Verification items for the finished model (mm, model axes). Face numbers are marked on the shaded views. Give positions to 0.01 mm unless a question says otherwise; leave off trailing zeros. Order: outer loops, then holes, each group sorted by start corner. A loop starts at its lowest first (then second) coordinate and runs counter-clockwise, first axis right, second up.
from build123d import *

# Parameters (mm, degrees)
BOSS_EXTRUDE1_DEPTH = 50
CUT_EXTRUDE2_START  = -63.5
SKETCH3_W           = 20
SKETCH3_H           = 10
CUT_EXTRUDE2_DEPTH  = 64.5
SKETCH4_W           = 17.5
SKETCH4_H           = 7
CUT_EXTRUDE3_DEPTH  = 10
BOSS_EXTRUDE2_DEPTH = 10
CUT_EXTRUDE6_DEPTH  = 10
SKETCH16_R          = 1.5
CUT_EXTRUDE7_DEPTH  = 10
SKETCH17_R          = 1.5
CUT_EXTRUDE8_DEPTH  = 10
CUT_EXTRUDE9_START  = -10
SKETCH18_R          = 1.5
CUT_EXTRUDE9_DEPTH  = 137
SKETCH19_R          = 1.5
CUT_EXTRUDE10_DEPTH = 10


with BuildPart() as part:
    # Sketch1 → Boss-Extrude1 (new body)
    with BuildSketch(Plane.XY):
        with BuildLine():
            ThreePointArc((59.5, 0), (0, -59.5), (-59.5, 0))
            Line((-59.5, 0), (-62.5, 0))
            ThreePointArc((-62.5, 0), (0, -62.5), (62.5, 0))
            Line((62.5, 0), (59.5, 0))
        make_face()
    extrude(amount=BOSS_EXTRUDE1_DEPTH)

    # Sketch3 → Cut-Extrude2 (cut)
    with BuildSketch(Plane(origin=(0, 0, 0), x_dir=(1, 0, 0), z_dir=(0, 1, 0)).offset(CUT_EXTRUDE2_START)):
        with Locations((-52.5, -45)):
            Rectangle(SKETCH3_W, SKETCH3_H)
        with Locations((52.5, -45)):
            Rectangle(SKETCH3_W, SKETCH3_H)
    cut_extrude2 = extrude(amount=CUT_EXTRUDE2_DEPTH, mode=Mode.SUBTRACT)

    # Sketch4 → Cut-Extrude3 (cut)
    with BuildSketch(Plane.XY.offset(50)):
        with Locations((0, -62.5)):
            Rectangle(SKETCH4_W, SKETCH4_H)
    cut_extrude3 = extrude(amount=-CUT_EXTRUDE3_DEPTH, mode=Mode.SUBTRACT)

    # Sketch9 → Boss-Extrude2 (add)
    with BuildSketch(Plane.XY):
        with BuildLine():
            Line((-52.112697755, -24.30055005), (-55.284775009, -25.779713966))
            ThreePointArc((-55.284775009, -25.779713966), (-51.730933866, -32.325075118), (-47.405903649, -38.388543854))
            Line((-47.405903649, -38.388543854), (-44.685892784, -36.185922485))
            ThreePointArc((-44.685892784, -36.185922485), (-48.762765529, -30.470357693), (-52.112697755, -24.30055005))
        make_face()
        with BuildLine():
            ThreePointArc((47.405903649, -38.388543854), (51.730933866, -32.325075118), (55.284775009, -25.779713966))
            Line((55.284775009, -25.779713966), (52.112697755, -24.30055005))
            ThreePointArc((52.112697755, -24.30055005), (48.762765529, -30.470357693), (44.685892784, -36.185922485))
            Line((44.685892784, -36.185922485), (47.405903649, -38.388543854))
        make_face()
        with BuildLine():
            Line((-7.007487246, -57.071403719), (-7.434029948, -60.54531525))
            ThreePointArc((-7.434029948, -60.54531525), (0, -61), (7.434029948, -60.54531525))
            Line((7.434029948, -60.54531525), (7.007487246, -57.071403719))
            ThreePointArc((7.007487246, -57.071403719), (0, -57.5), (-7.007487246, -57.071403719))
        make_face()
    boss_extrude2 = extrude(amount=BOSS_EXTRUDE2_DEPTH)

    # Sketch15 → Cut-Extrude6 (cut)
    with BuildSketch(Plane.XY):
        with BuildLine():
            Line((-52.112697755, -24.30055005), (-55.284775009, -25.779713966))
            ThreePointArc((-55.284775009, -25.779713966), (-51.730933866, -32.325075118), (-47.405903649, -38.388543854))
            Line((-47.405903649, -38.388543854), (-44.685892784, -36.185922485))
            ThreePointArc((-44.685892784, -36.185922485), (-48.762765529, -30.470357693), (-52.112697755, -24.30055005))
        make_face()
        with BuildLine():
            Line((-7.007487246, -57.071403719), (-7.434029948, -60.54531525))
            ThreePointArc((-7.434029948, -60.54531525), (0, -61), (7.434029948, -60.54531525))
            Line((7.434029948, -60.54531525), (7.007487246, -57.071403719))
            ThreePointArc((7.007487246, -57.071403719), (0, -57.5), (-7.007487246, -57.071403719))
        make_face()
        with BuildLine():
            ThreePointArc((47.405903649, -38.388543854), (51.730933866, -32.325075118), (55.284775009, -25.779713966))
            Line((55.284775009, -25.779713966), (52.112697755, -24.30055005))
            ThreePointArc((52.112697755, -24.30055005), (48.762765529, -30.470357693), (44.685892784, -36.185922485))
            Line((44.685892784, -36.185922485), (47.405903649, -38.388543854))
        make_face()
    cut_extrude6 = extrude(amount=CUT_EXTRUDE6_DEPTH, mode=Mode.SUBTRACT)

    # Sketch16 → Cut-Extrude7 (cut, symmetric)
    with BuildSketch(Plane(origin=(-28.846172405, -52.039872575, 0), x_dir=(0.874619707, -0.48480962, 0), z_dir=(0.48480962, 0.874619707, 0))):
        with Locations((-0.663731696, -45)):
            Circle(SKETCH16_R)
    cut_extrude7 = extrude(amount=CUT_EXTRUDE7_DEPTH, both=True, mode=Mode.SUBTRACT)

    # Sketch17 → Cut-Extrude8 (cut, symmetric)
    with BuildSketch(Plane(origin=(28.846172405, -52.039872575, 0), x_dir=(0.874619707, 0.48480962, 0), z_dir=(-0.48480962, 0.874619707, 0))):
        with Locations((0.663731696, -45)):
            Circle(SKETCH17_R)
    cut_extrude8 = extrude(amount=CUT_EXTRUDE8_DEPTH, both=True, mode=Mode.SUBTRACT)

    # Sketch18 → Cut-Extrude9 (cut)
    with BuildSketch(Plane(origin=(59.5, 0, 0), x_dir=(0, 1, 0), z_dir=(-1, 0, 0)).offset(CUT_EXTRUDE9_START)):
        with Locations((-6, -31)):
            Circle(SKETCH18_R)
    cut_extrude9 = extrude(amount=CUT_EXTRUDE9_DEPTH, mode=Mode.SUBTRACT)

    # Sketch19 → Cut-Extrude10 (cut, symmetric)
    with BuildSketch(Plane(origin=(0, -59.5, 0), x_dir=(1, 0, 0), z_dir=(0, 1, 0))):
        with Locations((0, -31)):
            Circle(SKETCH19_R)
    cut_extrude10 = extrude(amount=CUT_EXTRUDE10_DEPTH, both=True, mode=Mode.SUBTRACT)

    # Mirror4: Cut-Extrude2, Cut-Extrude3, Boss-Extrude2, Cut-Extrude6, Cut-Extrude7, Cut-Extrude8, Cut-Extrude9, Cut-Extrude10 across plane
    add(cut_extrude2.mirror(Plane.XY.offset(25)), mode=Mode.SUBTRACT)
    add(cut_extrude3.mirror(Plane.XY.offset(25)), mode=Mode.SUBTRACT)
    add(boss_extrude2.mirror(Plane.XY.offset(25)))
    add(cut_extrude6.mirror(Plane.XY.offset(25)), mode=Mode.SUBTRACT)
    add(cut_extrude7.mirror(Plane.XY.offset(25)), mode=Mode.SUBTRACT)
    add(cut_extrude8.mirror(Plane.XY.offset(25)), mode=Mode.SUBTRACT)
    add(cut_extrude9.mirror(Plane.XY.offset(25)), mode=Mode.SUBTRACT)
    add(cut_extrude10.mirror(Plane.XY.offset(25)), mode=Mode.SUBTRACT)


solid = part.part
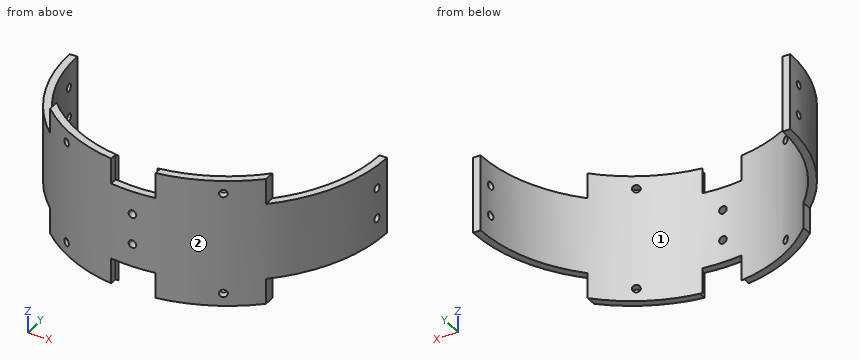
(1) Scan lines: line 1 (Z direction, x = 61.45, y = -6); line 2 (X direction, y = -30.5, z = 38.5); line 3 (X direction, y = -4, z = 25). Record each from-to range of solid material in increasing order.
Solved:
line 1: z = 10 to 17.5, 20.5 to 29.5, 32.5 to 40
line 2: x = -54.55 to -51.09, 51.09 to 54.55
line 3: x = -62.37 to -59.37, 59.37 to 62.37
(2) Go/stop test with flat-tipped pins: pin 1 (8 mm diameter, centred on x = -11, z = 30, fed in from +Y); pin 2 (5 mm diameter, centred on x = -5, z = 26, fed in from -Y); pin 3 (4 mm diameter, centred on y = -55.5, z = 13, fed in from -X); pin 4 (2.5 mm diameter, centred on x = 0, z = 19, fed in from -Y). Record where each tip stops, or that it passes through.
Solved:
pin 1: stops at y = -57.58
pin 2: stops at y = -62.45
pin 3: stops at x = -32.31
pin 4: passes through
(3) Section check D-D, the plane y = -44. Enter the section's corners in (x, z), then the cut area to 3 significant figures.
Solved:
outline: (-44.39, 10) - (-42.5, 10) - (-42.5, 0) - (-40.05, 0) - (-40.05, 50) - (-42.5, 50) - (-42.5, 40) - (-44.39, 40) - close; (40.05, 0) - (42.5, 0) - (42.5, 10) - (44.39, 10) - (44.39, 40) - (42.5, 40) - (42.5, 50) - (40.05, 50) - close
area: 358 mm2
(4) Section check C-C, the plane y = -6. Enter the section's corners in (x, z).
Solved:
outline: (-62.21, 10) - (-59.2, 10) - (-59.2, 17.5) - (-62.21, 17.5) - close; (-62.21, 20.5) - (-59.2, 20.5) - (-59.2, 29.5) - (-62.21, 29.5) - close; (-62.21, 32.5) - (-59.2, 32.5) - (-59.2, 40) - (-62.21, 40) - close; (59.2, 10) - (62.21, 10) - (62.21, 17.5) - (59.2, 17.5) - close; (59.2, 20.5) - (62.21, 20.5) - (62.21, 29.5) - (59.2, 29.5) - close; (59.2, 32.5) - (62.21, 32.5) - (62.21, 40) - (59.2, 40) - close
(5) Section check B-B, the plane z = 19. Enter the section's corners in (x, y).
Solved:
outline: (-62.5, 0) arc R62.5 ccw to (-62.34, -4.5) - (-59.33, -4.5) arc R59.5 cw to (-59.5, 0) - close; (-62.05, -7.5) arc R62.5 ccw to (-1.5, -62.48) - (-1.5, -59.48) arc R59.5 cw to (-59.03, -7.5) - close; (1.5, -62.48) arc R62.5 ccw to (62.05, -7.5) - (59.03, -7.5) arc R59.5 cw to (1.5, -59.48) - close; (59.33, -4.5) - (62.34, -4.5) arc R62.5 ccw to (62.5, 0) - (59.5, 0) arc R59.5 cw to start
(6) Section check A-A, the plane x = 0. Enter the section's corners in (y, z), then the cut area to 3 significant figures.
Solved:
outline: (-62.5, 10) - (-59.5, 10) - (-59.5, 17.5) - (-62.5, 17.5) - close; (-62.5, 20.5) - (-59.5, 20.5) - (-59.5, 29.5) - (-62.5, 29.5) - close; (-62.5, 32.5) - (-59.5, 32.5) - (-59.5, 40) - (-62.5, 40) - close
area: 72.0 mm2
(7) Release check for a two-part mould opening along X. For the marked faces 1 and 2 record: pulls with the +X half, pulls with the -X half, needs draft (parallel to the pull), parting line crosses it, or undercut.
Solved:
face 1: undercut
face 2: parting line crosses it
